```python
from build123d import *

# Parameters (mm, degrees)
SKETCH1_R               = 9
BOSS_EXTRUDE1_DEPTH     = 4
SKETCH2_R               = 5.9
BOSS_EXTRUDE2_DEPTH     = 20
CUT_EXTRUDE1_DEPTH      = 28.166155414
CUT_EXTRUDE1_DEPTH_BACK = 28.166155414
SKETCH4_R               = 0.425
CUT_EXTRUDE2_DEPTH      = 1.5


with BuildPart() as part:
    # Sketch1 → Boss-Extrude1 (new body)
    with BuildSketch(Plane(origin=(0, 0, 0), x_dir=(1, 0, 0), z_dir=(0, 1, 0))):
        with Locations(Location((0, 0, 0), (0, 0, 270))):
            Circle(SKETCH1_R)
    extrude(amount=BOSS_EXTRUDE1_DEPTH)

    # Sketch2 → Boss-Extrude2 (add)
    with BuildSketch(Plane(origin=(0, 4, 0), x_dir=(1, 0, 0), z_dir=(0, 1, 0))):
        with Locations(Location((0, 0, 0), (0, 0, 270))):
            Circle(SKETCH2_R)
    extrude(amount=BOSS_EXTRUDE2_DEPTH)

    # Sketch3 → Cut-Extrude1 (cut, two sides: drawn at the far end of the back side and taken through both)
    with BuildSketch(Plane(origin=(0, 0, 0), x_dir=(0, 0, -1), z_dir=(1, 0, 0)).offset(-CUT_EXTRUDE1_DEPTH_BACK)):
        Polygon((-6.28, 8.92), (6.28, 21.48), (6.28, 28.771900514), (-6.28, 28.771900514), align=None)
    extrude(amount=CUT_EXTRUDE1_DEPTH + CUT_EXTRUDE1_DEPTH_BACK, mode=Mode.SUBTRACT)

    # Sketch4 → Cut-Extrude2 (cut)
    with BuildSketch(Plane.XZ):
        with Locations(Location((0, -6, 0), (0, 0, 270))):
            Circle(SKETCH4_R)
    extrude(amount=-CUT_EXTRUDE2_DEPTH, mode=Mode.SUBTRACT)


solid = part.part
```
Design review of the part built by this model. Coordinates are the model's own, in mm. A direction names the side the tool comes from. Coordinates: 2 decimals unless noted, no trailing zeros. Loops run counter-clockwise (first coordinate to the right, second up) from the corner with the lowest first, then second, coordinate; pieces in that order, holes last. Notation, with made-up numbers: (-22, 76) -> (33, 76) arc R21 cw to (33, 109) -> close; hole circle Ø4 at (74, 28). An arc over 180 degrees is marked (long way). Answer as a JSON object with one key per item and string values.
Q1. Take a section at C-C on y = 4.5. Give the boundary of the cut face in (x, z).
Answer block:
{"outline": "circle Ø11.8 at (0, 0)"}
Q2. To check wall thickness, follow L1, parallel to Y at x = 6, z = 4.25; L2, parallel to X at y = 0.45, z = -6 (3 decimals); L3, parallel to Y at x = -1.75, z = -2.5. State the ranges of each line that lie inside material, in increasing order.
Answer block:
{"L1": "y = 0 to 4", "L2": "x = -6.708 to -0.425, 0.425 to 6.708", "L3": "y = 0 to 17.7"}
Q3. Take a section at B-B on x = 0. Give the boundary of the cut face in (y, z) (3 decimals), plus the area to 3 significant figures.
Answer block:
{"outline": "(0, -9) -> (4, -9) -> (4, -5.9) -> (21.1, -5.9) -> (9.3, 5.9) -> (4, 5.9) -> (4, 9) -> (0, 9) -> (0, -5.575) -> (1.5, -5.575) -> (1.5, -6.425) -> (0, -6.425) -> close", "area": "203 mm^2"}
Q4. Tool access review of faces 1 (the flat face through (0, 1.5, -6)), 2 (the cylindrical face through (2.703, 1.972, 8.584)): name each direction out of +Z, -Z, +X, -X, +Y, -Y from which nothing blocks a thin tool from reaching the whole face with its end or side.
Answer block:
{"face 1": "-Y", "face 2": "+Y, -Y"}
Q5. Take a section at A-A on z = 0. Give the boundary of the cut face in (x, y).
Answer block:
{"outline": "(-9, 0) -> (9, 0) -> (9, 4) -> (5.9, 4) -> (5.9, 15.2) -> (-5.9, 15.2) -> (-5.9, 4) -> (-9, 4) -> close"}
Q6. Take a section at D-D on x = 3. Give the boundary of the cut face in (y, z), plus the area to 3 significant figures.
Answer block:
{"outline": "(0, -8.49) -> (4, -8.49) -> (4, -5.08) -> (20.28, -5.08) -> (10.12, 5.08) -> (4, 5.08) -> (4, 8.49) -> (0, 8.49) -> close", "area": "182 mm^2"}
Q7. The part is to be moulded in two halves that separate along X. For faces 3 (the cylindrical face through (-0.163, 0.74, -6.393)), 4 (the cylindrical face through (0.259, 10.624, -5.894)), 5 (the flat face through (-6, 4, 2)), say which applies: +X half, -X half, draft (parallel to the pull), parting line (faces both ways), or undercut.
Answer block:
{"face 3": "undercut", "face 4": "parting line", "face 5": "draft"}
Q8. Clearance check with flat-ended pins moving along their axes: pin 1 Ø0.7 at (x, z) = (0, -6) entering from -Y; pin 2 Ø4 at (x, z) = (6, 0) entering from +Y; pin 3 Ø1.5 at (x, y) = (6, 15.5) entering from -Z. State where each tip first meets the part, or that it passes through.
Answer block:
{"pin 1": "stops at y = 1.5", "pin 2": "stops at y = 17.15", "pin 3": "stops at z = -2.69"}
